CAD build for the part. Positions are in the model's coordinates, mm. A direction names the side the tool comes from. Round coordinates to 2 decimals unless told otherwise and drop trailing zeros. Order: outer loops, then holes, each group sorted by start corner. A loop starts at its lowest first (then second) coordinate and runs counter-clockwise, first axis right, second up. Notation, with made-up numbers: M 70,82 L 100,82 A30 ccw 100,111 Z; hole C 85.25,-35 d10. An arc over 180 degrees is marked long. Answer as a JSON object with one key per item and string values.
```python
from build123d import *

# Parameters (mm, degrees)
BOSS_EXTRUDE1_DEPTH = 85
SKETCH6_R           = 0.501484151
CUT_EXTRUDE1_DEPTH  = 86
SKETCH7_R           = 0.300235793
BOSS_EXTRUDE2_DEPTH = 0.5
LPATTERN1_COUNT     = 9
LPATTERN1_PITCH     = 10


with BuildPart() as part:
    # Sketch5 → Boss-Extrude1 (new body)
    with BuildSketch(Plane(origin=(0, 0, 0), x_dir=(1, 0, 0), z_dir=(0, 1, 0))):
        Polygon((0, 16.765910013), (0, -34.714089987), (-6, -36.897911392), (-5.657979857, -37.837604013), (1.219310648, -35.334474977), (1.219310648, 16.765910013), align=None)
    extrude(amount=BOSS_EXTRUDE1_DEPTH)

    # Sketch6 → Cut-Extrude1 (cut, through all)
    with BuildSketch(Plane(origin=(0, 85, 0), x_dir=(1, 0, 0), z_dir=(0, 1, 0))):
        with Locations((0.617040076, 16.161484854)):
            Circle(SKETCH6_R)
    extrude(amount=-CUT_EXTRUDE1_DEPTH, mode=Mode.SUBTRACT)

    # Sketch7 → Boss-Extrude2 (add)
    with BuildSketch(Plane(origin=(11.156893463, 0, 30.65331286), x_dir=(-0.939692621, 0, 0.342020143), z_dir=(-0.342020143, 0, -0.939692621))):
        with Locations((16.976051075, 83.790382872)):
            Circle(SKETCH7_R)
    boss_extrude2 = extrude(amount=BOSS_EXTRUDE2_DEPTH)

    # Sketch10 → Revolve1 (revolve)
    with BuildSketch(Plane(origin=(-13.67960191, -0.418101739, 4.978967912), x_dir=(0.341719597, 0.010444277, 0.939743919), z_dir=(-0.939305295, -0.028708816, 0.341879168))):
        Polygon((33.002180094, 84.203214447), (33.002180094, 83.902962264), (32.435969012, 83.908878691), align=None)
    revolve1 = revolve(axis=Axis((-4.965313546, 83.790382872, 35.992565984), (-0.342020143, 0, -0.939692621)))

    # LPattern1: Boss-Extrude2, Revolve1 ×9
    with Locations(*[(0, -i * LPATTERN1_PITCH, 0) for i in range(1, LPATTERN1_COUNT)]):
        add(boss_extrude2)
        add(revolve1)


solid = part.part
```
Item 1: Saw through at C-C on x = -1.25. List the corners of the cut face in (y, z), and give its area (3 significant figures).
Worked answers:
{"outline": "M 0,35.17 L 85,35.17 L 85,36.23 L 0,36.23 Z", "area": "90.5 mm2"}
Item 2: Wall check: line 1 along X through (y, z) = (75.5, 27); line 2 along Z through (x, y) = (-2, 43); line 3 along Z through (x, y) = (-0.75, 73). Give the ranges that are in metal, low to high. Write a range as [from, to].
Worked answers:
{"line 1": "x = [0, 1.22]", "line 2": "z = [35.44, 36.51]", "line 3": "z = [34.99, 36.05]"}
Item 3: Saw through at A-A on y = 38.5. List the corners of the cut face in (x, z).
Worked answers:
{"outline": "M -6,36.9 L 0,34.71 L 0,-16.77 L 1.22,-16.77 L 1.22,35.33 L -5.66,37.84 Z; hole C 0.62,-16.16 d1"}
Item 4: Saw through at B-B on z = 6.5. List the corners of the cut face in (x, y), and give its area (3 significant figures).
Worked answers:
{"outline": "M 0,0 L 1.22,0 L 1.22,85 L 0,85 Z", "area": "104 mm2"}
Item 5: Drop flat-ended pins along their axis: pin 1 Ø15.5 at (y, z) = (61.5, 0.5) entering from -X; pin 2 Ø3 at (x, y) = (0.5, 53.5) entering from +Z. Give the stop position or say it passes through.
Worked answers:
{"pin 1": "stops at x = 0", "pin 2": "stops at z = 36.14"}
Item 6: 3-axis set-ups, long thin cutter, end or side, ignore diameter. For faces 1 (the flat face through (0.3, 0, 14.5)), 2 (the flat face through (0, 42, 9)): which of +Z, -Z, +X, -X, +Y, -Y reach the whole face in a straight line?
Worked answers:
{"face 1": "+Z, -Z, +X, -X, -Y", "face 2": "-Z, -X, +Y, -Y"}
